```python
from build123d import *

# Parameters (mm, degrees)
CYLINDER010_R     = 1.49
CYLINDER010_DEPTH = 10
ARRAY016_Y_COUNT  = 4
ARRAY016_Y_PITCH  = 7.58
BOX051_W          = 10
BOX051_H          = 10
BOX051_DEPTH      = 31
BOX050_W          = 10
BOX050_H          = 10
BOX050_DEPTH      = 30
BOX049_W          = 10
BOX049_H          = 10
BOX049_DEPTH      = 25
BOX048_W          = 10
BOX048_H          = 10
BOX048_DEPTH      = 25
BOX046_W          = 2
BOX046_H          = 80
BOX046_DEPTH      = 18
BOX047_W          = 4
BOX047_H          = 76
BOX047_DEPTH      = 18


with BuildPart() as array016:
    # Cylinder010 → Cylinder010 (new body)
    with BuildSketch(Plane(origin=(143, 6, 13), x_dir=(0, 0, -1), z_dir=(1, 0, 0))):
        Circle(CYLINDER010_R)
    extrude(amount=CYLINDER010_DEPTH)

    # Array016 Y: Array016 ×4


with BuildPart() as array016_1:
    add(array016.part)
    with Locations(*[(0, i * ARRAY016_Y_PITCH, 0) for i in range(1, ARRAY016_Y_COUNT)]):
        add(array016.part)


with BuildPart() as array016_2:
    # Array016 placement: moved
    add(array016_1.part.moved(Location((-33, 34.5, 0))))


with BuildPart() as obj1:
    # Box051 → Box051 (new body)
    with BuildSketch(Plane(origin=(110, 80.8, 0), x_dir=(1, 0, 0), z_dir=(0, 0, 1))):
        with Locations((5, 5)):
            Rectangle(BOX051_W, BOX051_H)
    extrude(amount=BOX051_DEPTH)


with BuildPart() as obj2:
    # Box050 → Box050 (new body)
    with BuildSketch(Plane(origin=(109, -8.8, 0), x_dir=(1, 0, 0), z_dir=(0, 0, 1))):
        with Locations((5, 5)):
            Rectangle(BOX050_W, BOX050_H)
    extrude(amount=BOX050_DEPTH)


with BuildPart() as obj3:
    # Box049 → Box049 (new body)
    with BuildSketch(Plane(origin=(114.8, 78.8, 0), x_dir=(1, 0, 0), z_dir=(0, 0, 1))):
        with Locations((5, 5)):
            Rectangle(BOX049_W, BOX049_H)
    extrude(amount=BOX049_DEPTH)


with BuildPart() as obj4:
    # Box048 → Box048 (new body)
    with BuildSketch(Plane(origin=(114.8, -6.8, 0), x_dir=(1, 0, 0), z_dir=(0, 0, 1))):
        with Locations((5, 5)):
            Rectangle(BOX048_W, BOX048_H)
    extrude(amount=BOX048_DEPTH)


with BuildPart() as obj5:
    # Box046 → Box046 (new body)
    with BuildSketch(Plane(origin=(113, 1, 23), x_dir=(1, 0, 0), z_dir=(0, 0, 1))):
        with Locations((1, 40)):
            Rectangle(BOX046_W, BOX046_H)
    extrude(amount=BOX046_DEPTH)


with BuildPart() as cut052:
    # Box047 → Box047 (new body)
    with BuildSketch(Plane(origin=(113, 3, 23), x_dir=(1, 0, 0), z_dir=(0, 0, 1))):
        with Locations((2, 38)):
            Rectangle(BOX047_W, BOX047_H)
    extrude(amount=BOX047_DEPTH)

    # Fusion008031: union obj5
    add(obj5.part)


with BuildPart() as cut052_1:
    # Fusion008031 placement: moved
    add(cut052.part.moved(Location((0, 0, -19))))

    # Cut047: cut obj4
    add(obj4.part, mode=Mode.SUBTRACT)

    # Cut048: cut obj3
    add(obj3.part, mode=Mode.SUBTRACT)

    # Cut049: cut obj2
    add(obj2.part, mode=Mode.SUBTRACT)

    # Cut050: cut obj1
    add(obj1.part, mode=Mode.SUBTRACT)

    # Cut052: cut Array016
    add(array016_2.part, mode=Mode.SUBTRACT)


solid = cut052_1.part
```
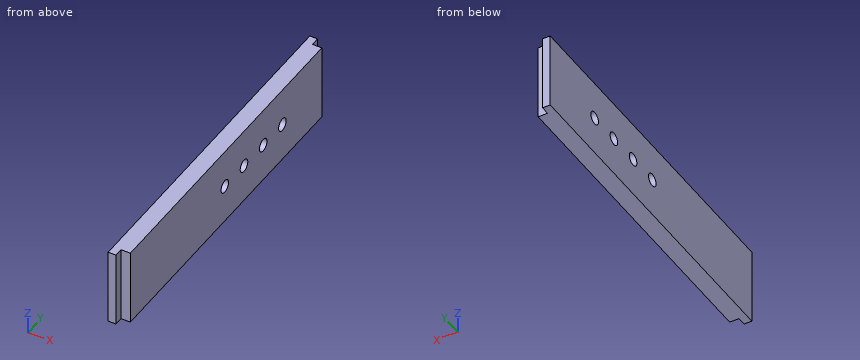
Check sheet for the modelled part. Datum: model origin and axes. Units: mm. Give positions to 0.01 mm unless a question says otherwise; leave off trailing zeros. Order: outer loops, then holes, each group sorted by start corner. A loop starts at its lowest first (then second) coordinate and runs counter-clockwise, first axis right, second up. Notation, with made-up numbers: M 43.5,60.25 L 79.5,60.25 A16 ccw 79.5,87.25 Z; hole C 2.25,28.5 d9. An arc over 180 degrees is marked long. Answer in a Markdown table with one row per item. Add a question column.
Q1. Gauge pin test, flat ends, axial feed: pin 1 Ø2 at (y, z) = (80, 17) entering from +X; pin 2 Ø1.1 at (x, z) = (116, 13) entering from +Y; pin 3 Ø0.7 at (x, z) = (116, 14.5) entering from -Y. Record the tip position at first contact, or that the pin passes through.
Q2. Sectioned sample at B-B, the plane x = 113.8. Record the boundary of the cut face in (y, z).
Q3. Sectioned sample at C-C, the plane z = 13. Record the boundary of the cut face in (x, y).
Q4. Sectioned sample at A-A, the plane y = 48.08. Record the boundary of the cut face in (x, z).
Q5. Sectioned sample at D-D, the plane z = 5. Record the boundary of the cut face in (x, y).
Q6. Thickness scan on L1, parallel to Y at x = 114.9, z = 13; L2, parallel to Y at x = 114.45, z = 13; L3, parallel to Z at x = 114.9, y = 55.66. Record the ranges inside material, lowest first.
Verdict:
| question | item | result |
|---|---|---|
| 1 | pin 1 | x = 114.8 |
| 1 | pin 2 | y = 78.8 |
| 1 | pin 3 | y = 3.2 |
| 2 | outline | M 1.2,4 L 80.8,4 L 80.8,22 L 1.2,22 Z; hole C 40.5,13 d2.98; hole C 48.08,13 d2.98; hole C 55.66,13 d2.98; hole C 63.24,13 d2.98 |
| 3 | outline | M 113,1.2 L 114.8,1.2 L 114.8,3.2 L 117,3.2 L 117,39.01 L 113,39.01 Z; M 113,41.99 L 117,41.99 L 117,46.59 L 113,46.59 Z; M 113,49.57 L 117,49.57 L 117,54.17 L 113,54.17 Z; M 113,57.15 L 117,57.15 L 117,61.75 L 113,61.75 Z; M 113,64.73 L 117,64.73 L 117,78.8 L 114.8,78.8 L 114.8,80.8 L 113,80.8 Z |
| 4 | outline | M 113,4 L 117,4 L 117,11.51 L 113,11.51 Z; M 113,14.49 L 117,14.49 L 117,22 L 113,22 Z |
| 5 | outline | M 113,1.2 L 114.8,1.2 L 114.8,3.2 L 117,3.2 L 117,78.8 L 114.8,78.8 L 114.8,80.8 L 113,80.8 Z |
| 6 | L1 | 3.2 to 39.01, 41.99 to 46.59, 49.57 to 54.17, 57.15 to 61.75, 64.73 to 78.8 |
| 6 | L2 | 1.2 to 39.01, 41.99 to 46.59, 49.57 to 54.17, 57.15 to 61.75, 64.73 to 80.8 |
| 6 | L3 | 4 to 11.51, 14.49 to 22 |
